The model under review builds one solid part; all positions refer to its coordinate system, in mm. Coordinates: 2 decimals unless noted, no trailing zeros. Order: outer loops, then holes, each group sorted by start corner. A loop starts at its lowest first (then second) coordinate and runs counter-clockwise, first axis right, second up. Notation, with made-up numbers: (-38.5, -39.75) -> (16.5, -39.75) arc R19 cw to (16.5, -22.75) -> close; hole circle Ø8 at (40.25, 78.5). An arc over 180 degrees is marked (long way). Use one line per item in the form item = value.
from build123d import *

# Parameters (mm, degrees)
SKETCH1_W           = 55
SKETCH1_H           = 8
BOSS_EXTRUDE1_DEPTH = 3
SKETCH2_R           = 1.7
CUT_EXTRUDE1_DEPTH  = 3
FILLET2_R           = 1
FILLET3_R           = 0.5
FILLET4_R           = 0.5


with BuildPart() as part:
    # Sketch1 → Boss-Extrude1 (new body)
    with BuildSketch(Plane(origin=(0, 0, 0), x_dir=(0, 1, 0), z_dir=(0, 0, 1))):
        Rectangle(SKETCH1_W, SKETCH1_H)
    extrude(amount=BOSS_EXTRUDE1_DEPTH)

    # Sketch2 → Cut-Extrude1 (cut)
    with BuildSketch(Plane.XY.offset(3)):
        with Locations((0, 21.5)):
            Circle(SKETCH2_R)
        with Locations((0, -21.5)):
            Circle(SKETCH2_R)
    extrude(amount=-CUT_EXTRUDE1_DEPTH, mode=Mode.SUBTRACT)

    # Fillet2
    fillet2_edges = [part.edges().sort_by_distance(p)[0] for p in [
        (0, 27.5, 3),
        (0, -27.5, 3),
    ]]
    fillet(fillet2_edges, radius=FILLET2_R)

    # Fillet3
    fillet3_edges = [part.edges().sort_by_distance(p)[0] for p in [
        (4, 0, 3),
        (-4, 0, 3),
        (4, 27.5, 1),
        (4, -27.5, 1),
        (4, 27.207106781, 2.707106781),
        (4, -27.207106781, 2.707106781),
        (-4, -27.5, 1),
        (-4, 27.5, 1),
        (-4, 27.207106781, 2.707106781),
        (-4, -27.207106781, 2.707106781),
    ]]
    fillet(fillet3_edges, radius=FILLET3_R)

    # Fillet4
    fillet4_edges = [part.edges().sort_by_distance(p)[0] for p in [
        (4, 0, 0),
        (0, -27.5, 0),
        (-4, 0, 0),
        (0, 27.5, 0),
        (-3.853553391, -27.353553391, 0),
        (-3.853553391, 27.353553391, 0),
        (3.853553391, 27.353553391, 0),
        (3.853553391, -27.353553391, 0),
    ]]
    fillet(fillet4_edges, radius=FILLET4_R)


solid = part.part
Item 1: Draft analysis for pull direction Y (two halves, no side actions). For faces 1 (the face through (-0.221, -19.814, 1.521)), 2 (the face through (0, 0, 0)), 3 (the face through (-0.049, 27.199, 2.715)), state which applies: released by +Y, released by -Y, zero draft, split by the parting line, or undercut.
Results found:
face_1 = undercut
face_2 = zero draft
face_3 = released by +Y
Item 2: We need section A-A (x = 0). Write out the cut boundary in (y, z), plus the area to 3 significant figures.
Results found:
outline = (-27.5, 0.5) arc R0.5 ccw to (-27, 0) -> (-23.2, 0) -> (-23.2, 3) -> (-26.5, 3) arc R1 ccw to (-27.5, 2) -> close; (-19.8, 0) -> (19.8, 0) -> (19.8, 3) -> (-19.8, 3) -> close; (23.2, 0) -> (27, 0) arc R0.5 ccw to (27.5, 0.5) -> (27.5, 2) arc R1 ccw to (26.5, 3) -> (23.2, 3) -> close
area = 144 mm²
Item 3: To check wall thickness, follow L1, parallel to Y at x = 0, z = 1.65; L2, parallel to Y at x = -1.25, z = 0.8; L3, parallel to Y at x = 3.25, z = 0.45. State the ranges of each line that lie inside material, in increasing order. Write a range as from..to.
Results found:
L1 = -27.5..-23.2, -19.8..19.8, 23.2..27.5
L2 = -27.5..-22.65, -20.35..20.35, 22.65..27.5
L3 = -27.5..27.5
Item 4: We need section B-B (y = 21.5). Write out the cut boundary in (x, z), plus the area to 3 significant figures.
Results found:
outline = (-4, 0.5) arc R0.5 ccw to (-3.5, 0) -> (-1.7, 0) -> (-1.7, 3) -> (-3.5, 3) arc R0.5 ccw to (-4, 2.5) -> close; (1.7, 0) -> (3.5, 0) arc R0.5 ccw to (4, 0.5) -> (4, 2.5) arc R0.5 ccw to (3.5, 3) -> (1.7, 3) -> close
area = 13.6 mm²
